from build123d import *


with BuildPart() as part:
    # Sketch1 → Revolve1 (revolve)
    with BuildSketch(Plane.XY):
        with BuildLine():
            Line((6, 0), (5, 0))
            Line((5, 0), (5, 5))
            Line((5, 5), (3.6, 5))
            Line((3.6, 5), (3.6, 14.5))
            Line((3.6, 14.5), (2, 14.5))
            Line((2, 14.5), (2, 15.117424305))
            ThreePointArc((2, 15.117424305), (3.001625132, 15.701219365), (3.841874542, 16.5))
            Line((3.841874542, 16.5), (4.6, 16.5))
            Line((4.6, 16.5), (4.6, 8.846468387))
            Line((4.6, 8.846468387), (6, 5))
            Line((6, 5), (6, 0))
        make_face()
    revolve(axis=Axis((0, 14.8, 0), (0, -1, 0)))


solid = part.part
Can you work these out from the model? Positions are in its coordinate system, mm. A direction names the side the tool comes from. Coordinates: 2 decimals unless noted, no trailing zeros. Write each loop counter-clockwise with the first axis right and the second up, starting at its lowest first coordinate (ties: lowest second). Pieces come first, ordered by that corner, then holes.
Q1. Imagine slicing it at D-D, the plane y = 3. List the corners of the cut face in (x, z) for me, plus the area to 3 significant figures.
Results found:
outline: circle Ø12 at (0, 0); hole circle Ø10 at (0, 0)
area: 34.6 mm2
Q2. Please list where these lines run through material, in increasing order: L1, parallel to Z at x = 0, y = 15.05; L2, parallel to Z at x = 0, y = 10.25; L3, parallel to Y at x = 4, z = 1.
Results found:
L1: z = -4.6 to -2, 2 to 4.6
L2: z = -4.6 to -3.6, 3.6 to 4.6
L3: y = 5 to 16.5
Q3. For P1, Ø6, axis at y = 8, z = 3.5, coming from the +X side; P2, Ø1, axis at y = 13, z = -2.5, coming from the +X side; P3, Ø5, axis at y = 5, z = -2, coming from the +X side; P4, Ø3, axis at x = 2, z = -2, coming from the -Y side, each with a flat end and sliding along its axis, tell me the tip position at first contact or that it passes through.
Results found:
P1: stops at x = 5.53
P2: stops at x = 4.14
P3: stops at x = 6
P4: stops at y = 5
Q4. Imagine slicing it at C-C, the plane y = 12. List the corners of the cut face in (x, z) for me, plus the area to 3 significant figures.
Results found:
outline: circle Ø9.2 at (0, 0); hole circle Ø7.2 at (0, 0)
area: 25.8 mm2
Q5. Which directions (+Z, -Z, +X, -X, +Y, -Y) give clear straight access to the entire face, cutting with the end or side of a thin tool? Please do faces 4 (the face through (3.434, 9.817, 1.081)), 5 (the face through (-0.434, 14.813, -1.952)), 6 (the face through (-3.65, 12.62, -2.8)).
Results found:
face 4: -Y
face 5: +Y, -Y
face 6: +Y
Q6. Imagine slicing it at B-B, the plane x = 0. List the corners of the cut face in (y, z) for me.
Results found:
outline: (0, -6) - (5, -6) - (8.85, -4.6) - (16.5, -4.6) - (16.5, -3.84) arc R5 cw to (15.12, -2) - (14.5, -2) - (14.5, -3.6) - (5, -3.6) - (5, -5) - (0, -5) - close; (0, 5) - (5, 5) - (5, 3.6) - (14.5, 3.6) - (14.5, 2) - (15.12, 2) arc R5 cw to (16.5, 3.84) - (16.5, 4.6) - (8.85, 4.6) - (5, 6) - (0, 6) - close
Q7. Imagine slicing it at A-A, the plane z = 0. List the corners of the cut face in (x, y) for me.
Results found:
outline: (-6, 0) - (-5, 0) - (-5, 5) - (-3.6, 5) - (-3.6, 14.5) - (-2, 14.5) - (-2, 15.12) arc R5 cw to (-3.84, 16.5) - (-4.6, 16.5) - (-4.6, 8.85) - (-6, 5) - close; (2, 14.5) - (3.6, 14.5) - (3.6, 5) - (5, 5) - (5, 0) - (6, 0) - (6, 5) - (4.6, 8.85) - (4.6, 16.5) - (3.84, 16.5) arc R5 cw to (2, 15.12) - close
Q8. If we mould it in two halves opening along X, with no side actions, what happens to faces 1 (the face through (-6, 2, 0)), 2 (the face through (-1.08, 2.54, -4.88)), 3 (the face through (1, 16.5, -4))? For each: +X half, -X half, draft (parallel to the pull), parting line (faces both ways), or undercut.
Results found:
face 1: parting line
face 2: undercut
face 3: draft
